Verification items for the finished model (mm, model axes). A direction names the side the tool comes from. Give positions to 0.01 mm unless a question says otherwise; leave off trailing zeros. Write each loop counter-clockwise with the first axis right and the second up, starting at its lowest first coordinate (ties: lowest second). Pieces come first, ordered by that corner, then holes. Notation, with made-up numbers: (22, 40.5) -> (66, 40.5) arc R17 cw to (66, 67.5) -> close; hole circle Ø10 at (-30, -29.75). An arc over 180 degrees is marked (long way). Use one line per item in the form item = value. Start each with the question number.
(1) Section check C-C, the plane y = 13. Record the cut outline in (x, z), plus the area to 3 significant figures.
(2) Scan lines: L1, parallel to X at y = 7.75, z = 6.5; L2, parallel to Z at x = -4, y = 17.25. Record each from-to range of solid material in increasing order.
(3) Set-up check for faces 1 (the face through (-0.2, 17.5, 13.25)), 2 (the face through (-12.5, 9, 0)), 3 (the face through (0, 9, 14)): record each of +Z, -Z, +X, -X, +Y, -Y from which the full face is reachable in a straight line by a thin tool's end or side.
(4) Section check A-A, the plane x = 3.75. Record the cut outline in (y, z).
(5) Depth check by flat-ended pin: pin 1 Ø12 at (x, z) = (4.5, -3.5) entering from -Y; pin 2 Ø12.5 at (x, z) = (-2, 5.5) entering from +Y. Enter the tip coordinate at first touch or a pass-through.
(6) Section check B-B, the plane z = -8.5. Record the cut outline in (x, y), plus the area to 3 significant figures.
(7) Release check for a two-part mould opening along X. For faces 4 (the face through (14, 9, 0)), 5 (the face through (0, 9, 12.5)), 6 (the face through (0, 1.5, 0)), 7 (the face through (-0.2, 17.5, -13.25)) record: pulls with the +X half, pulls with the -X half, needs draft (parallel to the pull), parting line crosses it, or undercut.
from build123d import *

# Parameters (mm, degrees)
SKETCH1_W           = 28
SKETCH1_H           = 28
BOSS_EXTRUDE1_DEPTH = 18
SHELL2_T            = -1.5
SKETCH2_W           = 26.5
SKETCH2_H           = 1
CUT_EXTRUDE1_DEPTH  = 29


with BuildPart() as part:
    # Sketch1 → Boss-Extrude1 (new body)
    with BuildSketch(Plane(origin=(0, 0, 0), x_dir=(1, 0, 0), z_dir=(0, 1, 0))):
        Rectangle(SKETCH1_W, SKETCH1_H)
    extrude(amount=BOSS_EXTRUDE1_DEPTH)

    # Shell2
    shell2_openings = [part.faces().sort_by_distance(p)[0] for p in [
        (0, 18, 0),
    ]]
    offset(amount=SHELL2_T, openings=shell2_openings, kind=Kind.INTERSECTION)

    # Sketch2 → Cut-Extrude1 (cut, through all)
    with BuildSketch(Plane.ZY.offset(14)):
        with Locations((0, 17.5)):
            Rectangle(SKETCH2_W, SKETCH2_H)
    extrude(amount=-CUT_EXTRUDE1_DEPTH, mode=Mode.SUBTRACT)


solid = part.part
Completed:
q1.outline = (-14, -14) -> (14, -14) -> (14, 14) -> (-14, 14) -> close; hole (-12.5, -12.5) -> (12.5, -12.5) -> (12.5, 12.5) -> (-12.5, 12.5) -> close
q1.area = 159 mm²
q2.L1 = -14 to -12.5, 12.5 to 14
q2.L2 = -14 to -13.25, 13.25 to 14
q3.face_1 = +X, -X, +Y
q3.face_2 = +Y
q3.face_3 = +Z, +X, -X, +Y, -Y
q4.outline = (0, -14) -> (18, -14) -> (18, -13.25) -> (17, -13.25) -> (17, -12.5) -> (1.5, -12.5) -> (1.5, 12.5) -> (17, 12.5) -> (17, 13.25) -> (18, 13.25) -> (18, 14) -> (0, 14) -> close
q5.pin_1 = 0
q5.pin_2 = 1.5
q6.outline = (-14, 0) -> (14, 0) -> (14, 17) -> (12.5, 17) -> (12.5, 1.5) -> (-12.5, 1.5) -> (-12.5, 17) -> (-14, 17) -> close
q6.area = 88.5 mm²
q7.face_4 = pulls with the +X half
q7.face_5 = undercut
q7.face_6 = undercut
q7.face_7 = needs draft
